from build123d import *

# Parameters (mm, degrees)
F2_R           = 2.54
F4_D           = 6.7564
F4_DEPTH       = 58.42
F4_CSINK_D     = 13.4874
F4_CSINK_ANGLE = 82
F4_TIP         = 2.0298273432
F6_D           = 4.2164
F6_DEPTH       = 18.2792094926


with BuildPart() as f1:
    # F0 (on Front) → F1 (revolve)
    with BuildSketch(Plane.XZ):
        Polygon((-52.7651011944, 8.2997372374), (-52.7651011944, 0), (58.0023080111, 0), (58.0023080111, 12.5073799863), (58.0023080111, 18.2782094926), (47.5186370313, 12.5073799863), (0, 12.5073799863), (-6.4646434039, 8.2997372374), align=None)
    revolve(axis=Axis((-11.7605924606, 0, 0), (1, 0, 0)))

    # F2
    f2_edges = [f1.edges().sort_by_distance(p)[0] for p in [
        (-52.765101, 0, -8.299737),
    ]]
    fillet(f2_edges, radius=F2_R)

    # F4
    with Locations(Plane.YZ.offset(58.0023080111)):
        with Locations((0, 0)):
            CounterSinkHole(F4_D / 2, F4_CSINK_D / 2, depth=F4_DEPTH, counter_sink_angle=F4_CSINK_ANGLE)
            with Locations((0, 0, -(F4_DEPTH + F4_TIP / 2))):  # 118° drill point
                Cone(0, F4_D / 2, F4_TIP, mode=Mode.SUBTRACT)

    # F6 (through all, one way)
    with BuildSketch(Plane(origin=(0, 0, 0), x_dir=(1, 0, 0), z_dir=(0, 0, -1))):
        with Locations((5.3260941058, 0)):
            Circle(F6_D / 2)
    extrude(amount=-F6_DEPTH, mode=Mode.SUBTRACT)


solid = f1.part
Verification items for the finished model (mm, model axes). A direction names the side the tool comes from. Coordinates: 2 decimals unless noted, no trailing zeros. Order: outer loops, then holes, each group sorted by start corner. A loop starts at its lowest first (then second) coordinate and runs counter-clockwise, first axis right, second up. Notation, with made-up numbers: M 38.25,88.25 L 60.25,88.25 A26 cw 60.25,104.25 Z; hole C 23.5,-26.5 d2. An arc over 180 degrees is marked long. One line per item, written item: value. Start each with the question number.
Item 1: Mould release check, pull along Y, two halves, no side actions. Record for faces 1 (the flat face through (58.002, 0, -8)), 2 (the conical face through (-2.095, -0.127, -0.573)), 3 (the conical face through (48.03, -3.84, 12.2)): released by +Y, released by -Y, zero draft, split by the parting line, or undercut.
Item 2: Sectioned sample at A-A (x = 31). Enter the section's corners in (y, z), then the cut area to 3 significant figures.
Item 3: Scan lines: probe 1 along Z at (x, y) = (43.5, 0); probe 2 along X at (y, z) = (0, 8.75). Record each from-to range of solid material in increasing order.
Item 4: Sectioned sample at C-C (x = 50.5). Enter the section's corners in (y, z), then the cut area to 3 significant figures.
Item 5: Access from +Z, -Z, +X, -X, +Y, -Y to the whole of each face (thin tool, end or side, straight path). Record for faces 4 (the cylindrical face through (23.43, -12.4, -1.63)), 5 (the cylindrical face through (5.05, -2.09, 7.5)), 6 (the cylindrical face through (26.475, 2.681, -2.056)), 7 (the flat face through (-52.765, 0, 0)).
Item 6: Sectioned sample at B-B (x = -9). Enter the section's corners in (y, z).
Item 7: Gauge pin test, flat ends, axial feed: pin 1 (6 mm diameter, centred on x = -33.5, y = 9.5, fed in from -Z); pin 2 (1 mm diameter, centred on y = 7.5, z = 11, fed in from -X); pin 3 (12 mm diameter, centred on x = -1, z = 4.5, fed in from +Y). Record the tip position at first contact, or that the pin passes through.
Conclusion:
1. face 1: zero draft
1. face 2: undercut
1. face 3: split by the parting line
2. outline: C 0,0 d25.01; hole C 0,0 d6.76
2. area: 456 mm^2
3. probe 1: z = -12.51 to -3.38, 3.38 to 12.51
3. probe 2: x = -5.77 to 3.22, 7.43 to 58
4. outline: C 0,0 d28.3; hole C 0,0 d6.76
4. area: 593 mm^2
5. face 4: -X
5. face 5: +Z
5. face 6: +X
5. face 7: +Z, -Z, -X, +Y, -Y
6. outline: C 0,0 d16.6
7. pin 1: stops at z = -5.16
7. pin 2: stops at x = 48.07
7. pin 3: stops at y = 12.51
